Geometry: final body of the model. Coordinates: model frame, mm. Face numbers are marked on the shaded views. A direction names the side the tool comes from. Round coordinates to 2 decimals unless told otherwise and drop trailing zeros. Write each loop counter-clockwise with the first axis right and the second up, starting at its lowest first coordinate (ties: lowest second). Pieces come first, ordered by that corner, then holes. Notation, with made-up numbers: M 35.25,-14 L 74.25,-14 A28 cw 74.25,16 Z; hole C -16.5,-0.5 d7. An arc over 180 degrees is marked long. Answer as CSV lines item,"result". Start each with the question number.
Q1. Ray query, probe 1 along X at (y, z) = (6.25, -0.75); probe 2 along Z at (x, y) = (2.5, 5); probe 3 along X at (y, z) = (-5.75, -0.7). Return the intervals inside material, ascending.
Q2. First-contact query: pin 1 (4.5 mm diameter, centred on x = -5, y = -3.5, fed in from -Z). Flat tip, straight axial feed; report the tip coordinate or a pass-through.
Q3. Mould query, pull axis Y, two halves, no side actions, for the marked faces 1 and 2. Classes: pulls with the +Y half, pulls with the -Y half, needs draft (parallel to the pull), parting line crosses it, or undercut.
Q4. Section query A-A on z = -0.85. Output: boundary loops of the cut face in (x, y), and give its area (3 significant figures).
Q5. Reachability of the marked faces 3 and 4 from +Z, -Z, +X, -X, +Y, -Y: full face, straight path, thin tool, end or side. Return the list, or none.
Q6. Section query D-D on y = 5. Output: boundary loops of the cut face in (x, z), and give its area (3 significant figures).
Q7. Section query B-B on x = -4. Output: boundary loops of the cut face in (y, z).
Q8. Section query C-C on y = -2.5. Output: boundary loops of the cut face in (x, z), and give its area (3 significant figures).
```python
from build123d import *

# Parameters (mm, degrees)
SALIENTE_EXTRUIR1_DEPTH = 1
SALIENTE_EXTRUIR2_DEPTH = 0.5


with BuildPart() as part:
    # Croquis1 → Saliente-Extruir1 (new body)
    with BuildSketch(Plane.XY):
        Polygon((5.877852523, -8.090169944), (9.510565163, 3.090169944), (0, 10), (-9.510565163, 3.090169944), (-5.877852523, -8.090169944), align=None)
        Polygon((9.040336961, 2.937383539), (0, 9.505572809), (-9.040336961, 2.937383539), (-5.587235512, -7.690169944), (5.587235512, -7.690169944), align=None, mode=Mode.SUBTRACT)
        Polygon((0.20966269, 9.353243948), (0, 9.505572809), (-0.210923368, 9.352328012), (-2.250282014, 3.090169944), (-8.830044516, 3.090169944), (-9.040336961, 2.937383539), (-8.960012395, 2.690169944), (-3.585831742, -1.214400854), (-5.664867685, -7.451242681), (-5.587235512, -7.690169944), (-5.318402678, -7.690169944), (-0.017323898, -3.899961523), (5.315095177, -7.690169944), (5.587235512, -7.690169944), (5.66389501, -7.454236269), (3.568710751, -1.226839982), (8.960012395, 2.690169944), (9.040336961, 2.937383539), (8.830044516, 3.090169944), (2.24, 3.090169944), align=None)
    extrude(amount=-SALIENTE_EXTRUIR1_DEPTH)

    # Croquis1_3 → Saliente-Extruir2 (add)
    with BuildSketch(Plane.XY):
        Polygon((8.830044516, 3.090169944), (0.20966269, 9.353243948), (2.24, 3.090169944), align=None)
        Polygon((-2.250282014, 3.090169944), (-0.210923368, 9.352328012), (-8.830044516, 3.090169944), align=None)
        Polygon((-3.585831742, -1.214400854), (-8.960012395, 2.690169944), (-5.664867685, -7.451242681), align=None)
        Polygon((-0.017323898, -3.899961523), (-5.318402678, -7.690169944), (5.315095177, -7.690169944), align=None)
        Polygon((5.66389501, -7.454236269), (8.960012395, 2.690169944), (3.568710751, -1.226839982), align=None)
    extrude(amount=-SALIENTE_EXTRUIR2_DEPTH)


solid = part.part
```
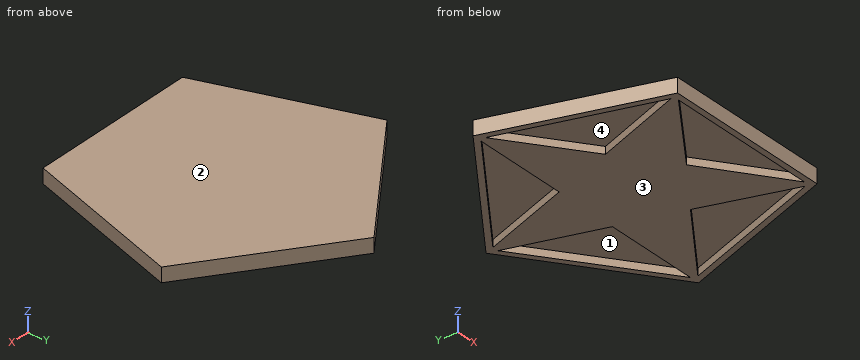
Entries:
1,probe 1,"x = -5.16 to -4.48, -1.22 to 1.22, 4.48 to 5.16"
1,probe 2,"z = -0.5 to 0"
1,probe 3,"x = -6.64 to -6.22, -5.1 to -2.6, 2.59 to 5.09, 6.22 to 6.64"
2,pin 1,"stops at z = -1"
3,face 1,"undercut"
3,face 2,"needs draft"
4,outline,"M -9.51,3.09 L -5.88,-8.09 L 5.88,-8.09 L 9.51,3.09 L 0,10 Z; hole M -8.96,2.69 L -5.66,-7.45 L -3.59,-1.21 Z; hole M -8.83,3.09 L -2.25,3.09 L -0.21,9.35 Z; hole M -5.32,-7.69 L 5.32,-7.69 L -0.02,-3.9 Z; hole M 0.21,9.35 L 2.24,3.09 L 8.83,3.09 Z; hole M 3.57,-1.23 L 5.66,-7.45 L 8.96,2.69 Z"
4,area,"135 mm^2"
5,face 3,"-Z, +X, -X, +Y, -Y"
5,face 4,"-Z"
6,outline,"M -6.88,-1 L -6.2,-1 L -6.2,-0.5 L -1.63,-0.5 L -1.63,-1 L 1.62,-1 L 1.62,-0.5 L 6.2,-0.5 L 6.2,-1 L 6.88,-1 L 6.88,0 L -6.88,0 Z"
6,area,"9.19 mm^2"
7,outline,"M -8.09,-1 L -7.69,-1 L -7.69,-0.5 L -6.75,-0.5 L -6.75,-1 L -2.46,-1 L -2.46,-0.5 L -0.91,-0.5 L -0.91,-1 L 3.09,-1 L 3.09,-0.5 L 6.6,-0.5 L 6.6,-1 L 7.09,-1 L 7.09,0 L -8.09,0 Z"
8,outline,"M -7.69,-1 L -7.27,-1 L -7.27,-0.5 L -4.01,-0.5 L -4.01,-1 L 4,-1 L 4,-0.5 L 7.27,-0.5 L 7.27,-1 L 7.69,-1 L 7.69,0 L -7.69,0 Z"
8,area,"12.1 mm^2"
